CAD build for the part. Positions are in the model's coordinates, mm. A direction names the side the tool comes from. Give positions to 0.01 mm unless a question says otherwise; leave off trailing zeros. Write each loop counter-clockwise with the first axis right and the second up, starting at its lowest first coordinate (ties: lowest second). Pieces come first, ordered by that corner, then holes. Notation, with made-up numbers: (19.25, 47) -> (63.25, 47) arc R19 cw to (63.25, 83) -> close; hole circle Ø3 at (23.25, -36). An arc over 180 degrees is marked (long way). Answer as a JSON object with one key per item and string values.
```python
from build123d import *

# Parameters (mm, degrees)
SKETCH_1_R          = 22.5
SKETCH_1_R_2        = 1.25
EXTRUDE_1_DEPTH     = 5
SKETCH_2_R          = 17.5
EXTRUDE_2_DEPTH     = 6
SKETCH_3_R          = 2
EXTRUDE_3_DEPTH     = 3.5
FILLET_1_R          = 0.5
FILLET_2_R          = 0.25
CUT_EXTRUDE_1_DEPTH = 3
SKETCH_5_R          = 7
CUT_EXTRUDE_2_DEPTH = 11
SKETCH_6_W          = 10.283159463
SKETCH_6_H          = 33.988548121
CUT_EXTRUDE_3_DEPTH = 17


with BuildPart() as part:
    # 草图1 → 凸台-拉伸1 (new body)
    with BuildSketch(Plane.XY):
        Circle(SKETCH_1_R)
        with Locations((0, 20)):
            Circle(SKETCH_1_R_2, mode=Mode.SUBTRACT)
        with Locations((0, -20)):
            Circle(SKETCH_1_R_2, mode=Mode.SUBTRACT)
        with Locations((-20, 0)):
            Circle(SKETCH_1_R_2, mode=Mode.SUBTRACT)
    extrude(amount=EXTRUDE_1_DEPTH)

    # 草图2 → 凸台-拉伸2 (add)
    with BuildSketch(Plane.XY.offset(5)):
        Circle(SKETCH_2_R)
    extrude(amount=EXTRUDE_2_DEPTH)

    # 草图3 → 凸台-拉伸3 (add)
    with BuildSketch(Plane.XY.offset(11)):
        with Locations((-9.367828489, 10.404027557)):
            Circle(SKETCH_3_R)
    extrude(amount=EXTRUDE_3_DEPTH)

    # 圆角1
    fillet_1_edges = [part.edges().sort_by_distance(p)[0] for p in [
        (-17.5, 0, 11),
    ]]
    fillet(fillet_1_edges, radius=FILLET_1_R)

    # 圆角2
    fillet_2_edges = [part.edges().sort_by_distance(p)[0] for p in [
        (-11.367828489, 10.404027557, 11),
        (-11.367828489, 10.404027557, 14.5),
    ]]
    fillet(fillet_2_edges, radius=FILLET_2_R)

    # 草图4 → 切除-拉伸1 (cut)
    with BuildSketch(Plane.XY.offset(11)):
        with BuildLine():
            ThreePointArc((-16.962482908, 6.022804462), (-8.539705078, -15.845297005), (14.357267915, -10.856742514))
            ThreePointArc((14.357267915, -10.856742514), (13.579373382, -5.253629085), (7.976259953, -6.031523619))
            ThreePointArc((7.976259953, -6.031523619), (-4.744280599, -8.802942781), (-9.423601616, 3.346002479))
            ThreePointArc((-9.423601616, 3.346002479), (-11.85464127, 8.453844117), (-16.962482908, 6.022804462))
        make_face()
    extrude(amount=-CUT_EXTRUDE_1_DEPTH, mode=Mode.SUBTRACT)

    # 草图5 → 切除-拉伸2 (cut)
    with BuildSketch(Plane.XY.offset(11)):
        Circle(SKETCH_5_R)
    extrude(amount=-CUT_EXTRUDE_2_DEPTH, mode=Mode.SUBTRACT)

    # 草图6 → 切除-拉伸3 (cut)
    with BuildSketch(Plane.XY.offset(5)):
        with Locations((24.941579731, -0.947133109)):
            Rectangle(SKETCH_6_W, SKETCH_6_H)
    extrude(amount=-CUT_EXTRUDE_3_DEPTH, mode=Mode.SUBTRACT)


solid = part.part
```
1) Slice it at C-C (y = -20). List the corners of the cut face in (x, z).
Model answer:
{"outline": "(-10.31, 0) -> (-1.25, 0) -> (-1.25, 5) -> (-10.31, 5) -> close; (1.25, 0) -> (10.31, 0) -> (10.31, 5) -> (1.25, 5) -> close"}
2) Pin check, flat tips, straight feed: pin 1 (8 mm diameter, centred on y = 17.5, z = 4.5, fed in from +X); pin 2 (6 mm diameter, centred on x = -2.5, y = 0.5, fed in from -Z); pin 3 (1.5 mm diameter, centred on x = 10.5, z = 9.5, fed in from +Y); pin 4 (3 mm diameter, centred on x = 0, y = 20, fed in from +Z). Stop position of each tip, or through.
Model answer:
{"pin 1": "stops at x = 18", "pin 2": "passes through", "pin 3": "stops at y = 14.53", "pin 4": "stops at z = 5"}
3) Slice it at A-A (x = 0). List the corners of the cut face in (y, z).
Model answer:
{"outline": "(-22.5, 0) -> (-21.25, 0) -> (-21.25, 5) -> (-22.5, 5) -> close; (-18.75, 0) -> (-7, 0) -> (-7, 11) -> (-10, 11) -> (-10, 8) -> (-17.5, 8) -> (-17.5, 5) -> (-18.75, 5) -> close; (7, 0) -> (18.75, 0) -> (18.75, 5) -> (17.5, 5) -> (17.5, 10.5) arc R0.5 ccw to (17, 11) -> (7, 11) -> close; (21.25, 0) -> (22.5, 0) -> (22.5, 5) -> (21.25, 5) -> close"}
4) 3-axis set-ups, long thin cutter, end or side, ignore diameter. For faces 1 (the flat face through (-9.3, 15.1, 5)), 2 (the cylindrical face through (-0.27, -21.22, 2.46)): which of +Z, -Z, +X, -X, +Y, -Y reach the whole face in a straight line?
Model answer:
{"face 1": "+Z", "face 2": "+Z, -Z"}
5) Slice it at B-B (y = 0). List the corners of the cut face in (x, z).
Model answer:
{"outline": "(-22.5, 0) -> (-21.25, 0) -> (-21.25, 5) -> (-22.5, 5) -> close; (-18.75, 0) -> (-7, 0) -> (-7, 11) -> (-10, 11) -> (-10, 8) -> (-17.5, 8) -> (-17.5, 5) -> (-18.75, 5) -> close; (7, 0) -> (19.8, 0) -> (19.8, 5) -> (17.5, 5) -> (17.5, 10.5) arc R0.5 ccw to (17, 11) -> (7, 11) -> close"}
6) Slice it at D-D (z = 1). List the corners of the cut face in (x, y).
Model answer:
{"outline": "(19.8, -10.69) -> (19.8, 10.69) arc R22.5 ccw (long way) to start; hole circle Ø2.5 at (-20, 0); hole circle Ø14 at (0, 0); hole circle Ø2.5 at (0, -20); hole circle Ø2.5 at (0, 20)"}
7) Wall check: probe 1 along Y at (x, z) = (0, 3.25); probe 2 along Z at (x, y) = (-10, 19); probe 3 along Z at (x, y) = (0, -7.5). Give the ranges that are in metal, low to high.
Model answer:
{"probe 1": "y = -22.5 to -21.25, -18.75 to -7, 7 to 18.75, 21.25 to 22.5", "probe 2": "z = 0 to 5", "probe 3": "z = 0 to 11"}
